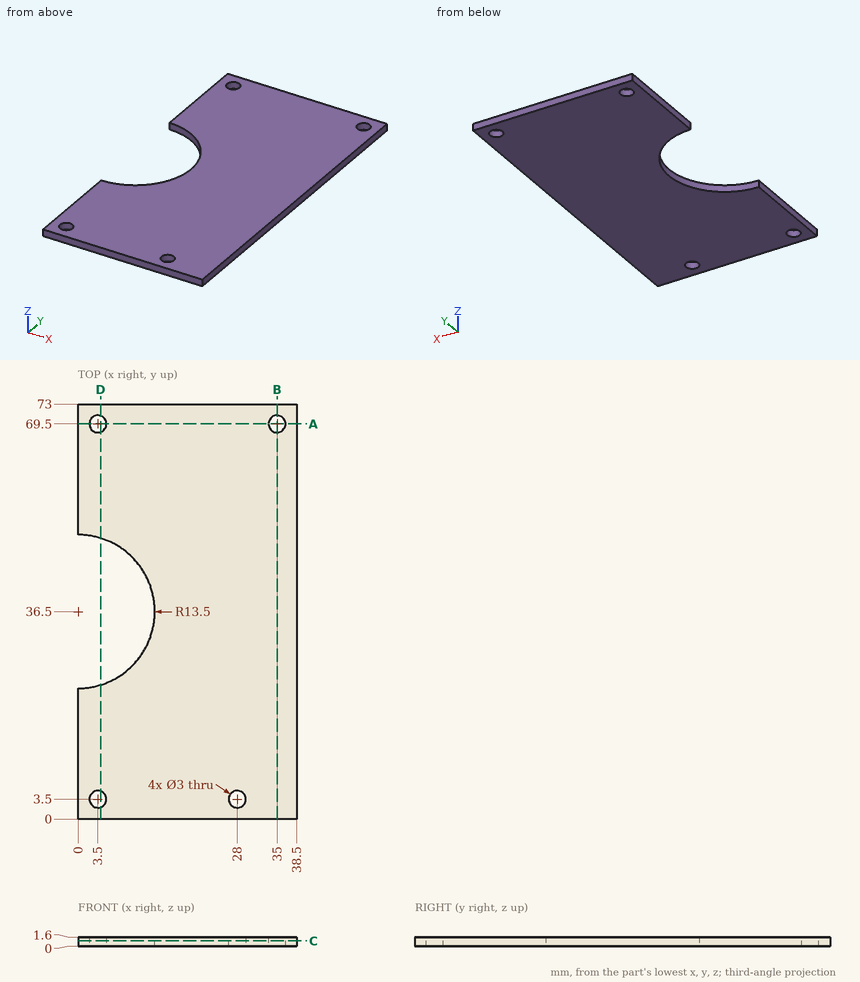
Job drawing, mm, ordinate dimensions from the low corner. One solid piece. Round coordinates to 2 decimals unless told otherwise and drop trailing zeros. Order: outer loops, then holes, each group sorted by start corner. A loop starts at its lowest first (then second) coordinate and runs counter-clockwise, first axis right, second up. Notation, with made-up numbers: M -18.5,34 L -13.5,34 A17 cw -13.5,67 Z; hole C 63,79 d11. An arc over 180 degrees is marked long. Write each question's results on one line, items separated by ' | '. Start each with the question number.
(1) Saw through at B-B, the plane x = 35. Give the cut face in (y, z), then the cut area to 3 significant figures.
(2) Saw through at C-C, the plane z = 0.95. Give the cut face in (x, y), then the cut area to 3 significant figures.
(3) Drop a flat-ended pin along its axis: pin 1 (2.5 mm diameter, centred on x = 28, y = 3.5, fed in from +Z). Give the stop position or say it passes through.
(4) Saw through at D-D, the plane x = 4. Give the cut face in (y, z).
(5) Saw through at A-A, the plane y = 69.5. Give the cut face in (x, z).
(6) Probe probe 1 along X at (y, z) = (69.5, 0.55); probe 2 along Y at (x, z) = (35, 0.95); probe 3 along Y at (x, z) = (3.5, 0.8). List the from-to ranges inside material, lowest first. Write a range as from..to.
Established:
1) outline: M 0,0 L 68,0 L 68,1.6 L 0,1.6 Z; M 71,0 L 73,0 L 73,1.6 L 71,1.6 Z | area: 112 mm^2
2) outline: M 0,0 L 38.5,0 L 38.5,73 L 0,73 L 0,50 A13.5 cw 0,23 Z; hole C 3.5,3.5 d3; hole C 3.5,69.5 d3; hole C 28,3.5 d3; hole C 35,69.5 d3 | area: 2,500 mm^2
3) pin 1: passes through
4) outline: M 0,0 L 2.09,0 L 2.09,1.6 L 0,1.6 Z; M 4.91,0 L 23.61,0 L 23.61,1.6 L 4.91,1.6 Z; M 49.39,0 L 68.09,0 L 68.09,1.6 L 49.39,1.6 Z; M 70.91,0 L 73,0 L 73,1.6 L 70.91,1.6 Z
5) outline: M 0,0 L 2,0 L 2,1.6 L 0,1.6 Z; M 5,0 L 33.5,0 L 33.5,1.6 L 5,1.6 Z; M 36.5,0 L 38.5,0 L 38.5,1.6 L 36.5,1.6 Z
6) probe 1: x = 0..2, 5..33.5, 36.5..38.5 | probe 2: y = 0..68, 71..73 | probe 3: y = 0..2, 5..23.46, 49.54..68, 71..73
